The listing builds one solid part. Answer for the finished solid, in the listing's coordinates (mm). Face numbers are marked on the shaded views. Give positions to 0.01 mm unless a question says otherwise; leave off trailing zeros. Write each loop counter-clockwise with the first axis right and the second up, starting at its lowest first coordinate (ties: lowest second). Pieces come first, ordered by that corner, then holes. Notation, with made-up numbers: (37, 1) - (48, 1) arc R18 cw to (48, 9) - close; hole circle Ø8 at (74, 13.25). An arc over 180 degrees is marked (long way). Answer in a Markdown table with one row per item. Add a question column.
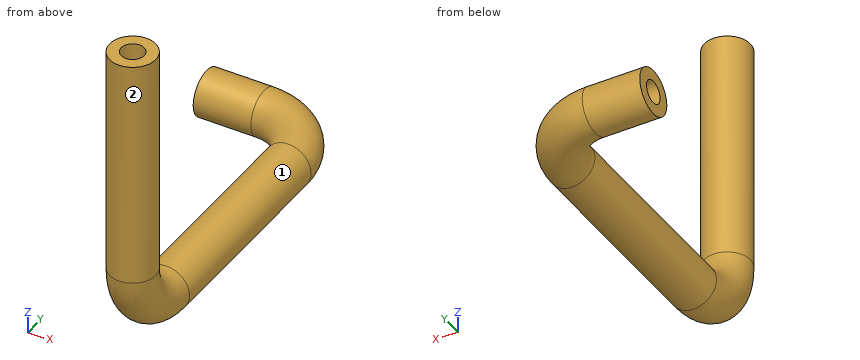
Autodesk Inventor part; units mm, degrees
ref_plane "YZ Plane" through (0, 0, 0) normal (1, 0, 0) x (0, 1, 0)
ref_plane "XZ Plane" through (0, 0, 0) normal (0, 1, 0) x (-1, 0, 0)
ref_plane "XY Plane" through (0, 0, 0) normal (0, 0, 1) x (1, 0, 0)
sketch "Sketch2" plane through (0, 0, 0) normal (1, 0, 0) x (0, 1, 0)
  circle A0 centre (0, 0) radius 1
  circle A1 centre (0, 0) radius 2
  dimension "d8" = 2
  dimension "d9" = 1
sketch3d "3D Sketch1"
  line L0 (0, 0, 0) -> (5, 0, 0)
  arc A0 (5, 0, 0) -> (10, -5, 0) centre (5, -5, 0) ccw
  line L1 (10, -5, 0) -> (10, -23, 0)
  arc A1 (10, -23, 0) -> (10, -28, 5) centre (10, -23, 5) ccw
  line L2 (10, -28, 5) -> (10, -28, 25)
  dimension "d3" = 10
  dimension "d4" = 28
  dimension "d6" = 5
  dimension "d12" = 25
  dimension "d13" = 5
sweep "Sweep1" add profiles "Sketch2" path "3D Sketch1"
properties part number "Pipe2"
1. Section B-B (y = -10.5) is taken. Give the vertices of the cut face in (x, z), and give its area (3 significant figures).
2. Given pin 1 Ø8 at (y, z) = (-19, 16) entering from +X; pin 2 Ø1.6 at (x, z) = (10, 0) entering from -Y; pin 3 Ø1 at (x, y) = (3.5, -2) entering from -Z; pin 4 Ø6 at (x, z) = (9, 7) entering from +Y, each flat-ended and moving along its own axis, determine where each tip first touches the part or whether it passes through.
3. The mould has two halves that part along Y. Classify the marked faces 1 and 2: +Y half, -Y half, draft (parallel to the pull), parting line (faces both ways), or undercut.
4. Straight lines are drawn through the part: L1, parallel to Z at x = 10, y = -19.5; L2, parallel to Y at x = 10, z = 13; L3, parallel to Y at x = 3.75, z = 0.25. For each, find the intervals that lie inside material, in ascending order. Write a range as [from, to].
5. Section A-A (z = 10.75) is taken. Give the vertices of the cut face in (x, y).
Geometry check:
| question | item | result |
|---|---|---|
| 1 | outline | circle Ø4 at (10, 0); hole circle Ø2 at (10, 0) |
| 1 | area | 9.42 mm² |
| 2 | pin 1 | through |
| 2 | pin 2 | y = -28.6 |
| 2 | pin 3 | z = -1.32 |
| 2 | pin 4 | y = -25.87 |
| 3 | face 1 | undercut |
| 3 | face 2 | parting line |
| 4 | L1 | [-2, -1], [1, 2] |
| 4 | L2 | [-30, -29], [-27, -26] |
| 4 | L3 | [-1.98, -0.97], [0.97, 1.98] |
| 5 | outline | circle Ø4 at (10, -28); hole circle Ø2 at (10, -28) |
